Could you check a few things on this model? Use its own coordinates, in mm. Give positions to 0.01 mm unless a question says otherwise; leave off trailing zeros. Write each loop counter-clockwise with the first axis right and the second up, starting at its lowest first coordinate (ties: lowest second). Pieces come first, ordered by that corner, then holes. Notation, with made-up numbers: M 58,52 L 74,52 A4 cw 74,58 Z; hole C 45,56 d4. An arc over 180 degrees is marked long. One line per item, written item: value.
```python
from build123d import *

# Parameters (mm, degrees)
F1_R     = 3.175
F3_W     = 304.8
F3_H     = 25.4
F4_DEPTH = 228.6


with BuildPart() as f2:
    # F2: sweep along a path in F0
    with BuildLine(Plane.XY) as f2_path:
        Line((228.9410829544, -232.7981889248), (228.9410829544, 156.5981889248))
        ThreePointArc((228.9410829544, 156.5981889248), (206.6226196808, 210.4797256512), (152.7410829544, 232.7981889248))
        Line((152.7410829544, 232.7981889248), (-152.7410829544, 232.7981889248))
        ThreePointArc((-152.7410829544, 232.7981889248), (-206.6226196808, 210.4797256512), (-228.9410829544, 156.5981889248))
        Line((-228.9410829544, 156.5981889248), (-228.9410829544, -232.7981889248))
    # F1 (on Front) → F2 (sweep)
    with BuildSketch(Plane.XZ):
        with Locations((-228.9410680532, 0)):
            Circle(F1_R)
    sweep(path=f2_path.line)

    # F3 (on Top) → F4 (join, symmetric)
    with BuildSketch(Plane.XY):
        with Locations((0, 233.5601756576)):
            Rectangle(F3_W, F3_H)
    extrude(amount=F4_DEPTH, both=True)


solid = f2.part
```
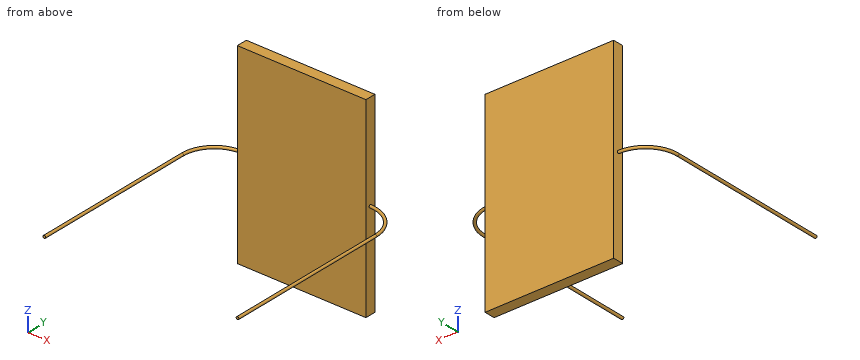
1) I'm going to push a flat-ended pin straight in: pin 1 (2 mm diameter, centred on x = 147.5, z = 147, fed in from -Y). Where does the tip first touch, or does it pass through?
Outcome:
pin 1: stops at y = 220.86
2) Please list where these lines run through material, in increasing order: L1, parallel to Y at x = 21, z = -78.5; L2, parallel to X at y = 225, z = 108. Write a range as from..to.
Outcome:
L1: y = 220.86..246.26
L2: x = -152.4..152.4
3) If we section it at B-B, the plane x = 109: Write out the boundary of the cut face in (y, z).
Outcome:
outline: M 220.86,-228.6 L 246.26,-228.6 L 246.26,228.6 L 220.86,228.6 Z
4) If we section it at A-A, the plane z = 82.5: Write out the boundary of the cut face in (x, y), then the cut area to 3 significant figures.
Outcome:
outline: M -152.4,220.86 L 152.4,220.86 L 152.4,246.26 L -152.4,246.26 Z
area: 7,740 mm^2
